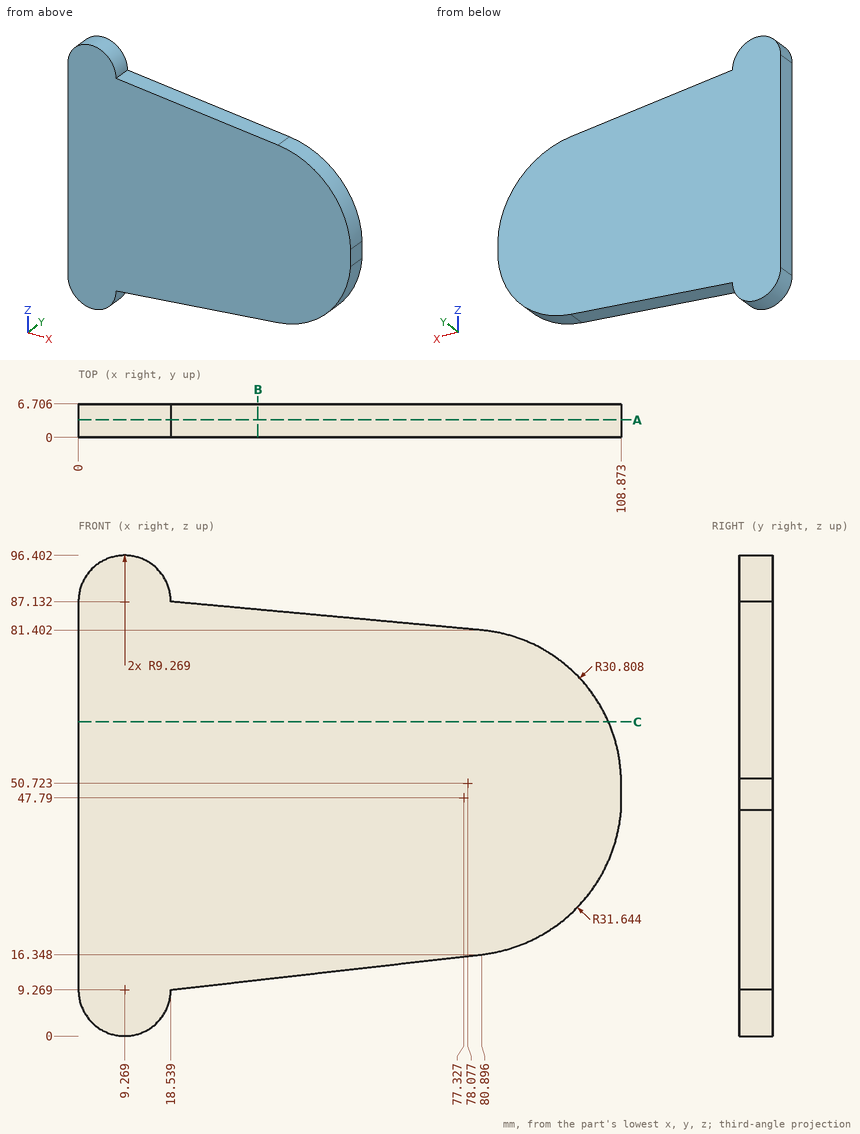
Study the drawing (mm; zero at the part's minimum x, y, z) and answer. Give positions to 0.01 mm unless a question says otherwise; leave off trailing zeros. Write each loop counter-clockwise with the first axis right and the second up, starting at its lowest first coordinate (ties: lowest second). Pieces come first, ordered by that corner, then holes. Notation, with made-up numbers: (53.5, 57.25) - (96.5, 57.25) arc R11 ccw to (96.5, 77.25) - close; hole circle Ø2 at (-14, 71.25). An arc over 180 degrees is marked (long way). One line per question, with ' | ' between items. Start each with the question number.
1. Straight lines are drawn through the part: line 1 (X direction, y = 4, z = 20) (1 decimal); line 2 (Z direction, x = 54, y = 1) (1 decimal); line 3 (Z direction, x = 69, y = 2) (1 decimal). For each, find the intervals that lie inside material, in ascending order.
2. Section B-B, the plane x = 36 is taken. Determine the outline of the cut face in (y, z) (1 decimal), then the cut area to 3 significant figures.
3. Section A-A, the plane y = 3.5 is taken. Determine the outline of the cut face in (x, z) (1 decimal).
4. Section C-C, the plane z = 63 is taken. Determine the outline of the cut face in (x, y) (1 decimal).
5. Given P1, Ø2, axis at x = 95, y = 6, coming from the -Z side (1 decimal), flat-ended and moving along its own axis, determine where the tip first touches the part or whether it passes through.
Result:
1) line 1: x = 0 to 92.5 | line 2: z = 13.3 to 83.9 | line 3: z = 15 to 82.5
2) outline: (0, 11.3) - (6.7, 11.3) - (6.7, 85.5) - (0, 85.5) - close | area: 498 mm2
3) outline: (0, 9.3) arc R9.3 ccw to (18.5, 9.3) - (80.9, 16.3) arc R31.6 ccw to (108.9, 45.3) - (108.9, 51.6) arc R30.8 ccw to (80.9, 81.4) - (18.5, 87.1) arc R9.3 ccw to (0, 87.1) - close
4) outline: (0, 0) - (106.3, 0) - (106.3, 6.7) - (0, 6.7) - close
5) P1: stops at z = 20.9
